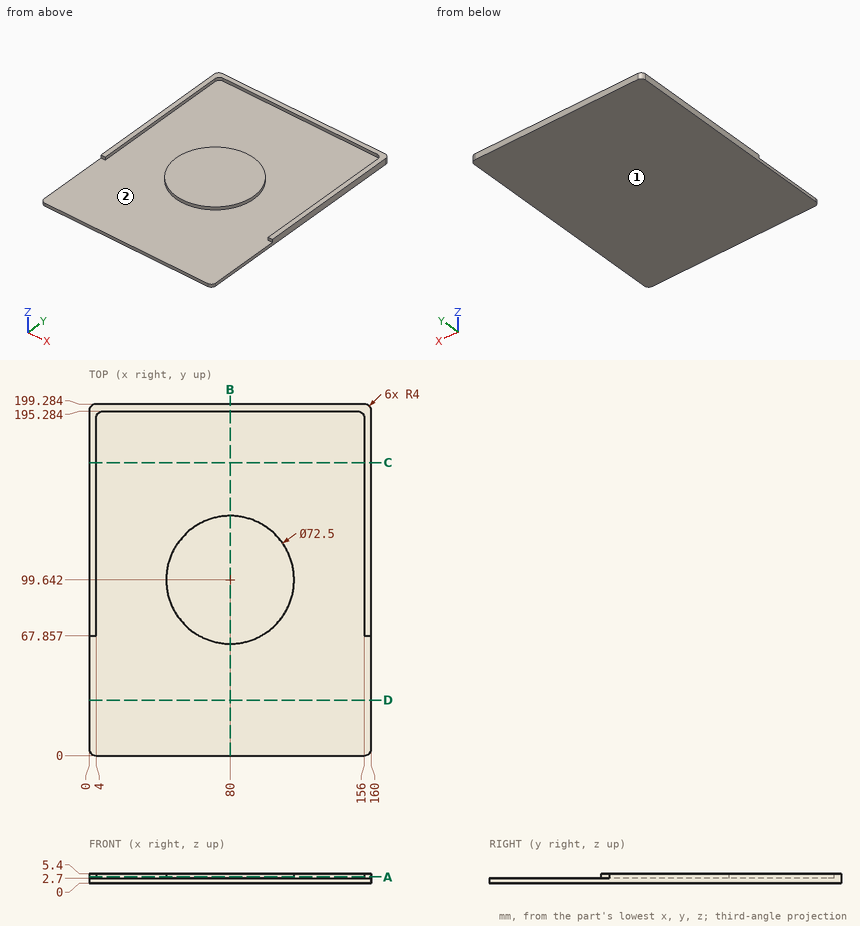
The figure shows three views and two pictorial views of one solid part (mm, origin at its lowest corner). Answer the questions. Round coordinates to 2 decimals unless told otherwise and drop trailing zeros. Loops run counter-clockwise (first coordinate to the right, second up) from the corner with the lowest first, then second, coordinate; pieces in that order, holes last. Notation, with made-up numbers: M 69,-23.75 L 89,-23.75 A19 ccw 89,-11.75 Z; hole C 20.5,-27 d4. An arc over 180 degrees is marked long. Write each question's results on one line, items separated by ' | '. Start each with the question number.
1) Find section B-B on x = 80. Write down the section's boundary in (y, z).
2) Each of these flat-tipped pins is pushed along its axis until it touches: pin 1 (1.4 mm diameter, centred on x = 68, z = 3.5, fed in from -Y); pin 2 (1.4 mm diameter, centred on x = 2, z = 4, fed in from -Y). Where does it stop, or does it pass through?
3) Find section C-C on y = 166. Write down the section's boundary in (x, z).
4) Find section A-A on z = 3.6. Write down the section's boundary in (x, y).
5) Find section D-D on y = 31.5. Write down the section's boundary in (x, z).
6) Determine the mould class of the marked faces 1 and 2 for opening direction X: pulls with the +X half, pulls with the -X half, needs draft (parallel to the pull), parting line crosses it, or undercut.
7) Straight lines are drawn through the part: probe 1 along X at (y, z) = (190.5, 3.35); probe 2 along X at (y, z) = (122, 2.75) (1 decimal); probe 3 along Z at (x, y) = (120.5, 116). For each, find the intervals that lie inside material, in ascending order.
Final values:
1) outline: M 0,0 L 199.28,0 L 199.28,5.4 L 195.28,5.4 L 195.28,2.7 L 135.89,2.7 L 135.89,5.4 L 63.39,5.4 L 63.39,2.7 L 0,2.7 Z
2) pin 1: y = 65.2 | pin 2: y = 67.86
3) outline: M 0,0 L 160,0 L 160,5.4 L 156,5.4 L 156,2.7 L 4,2.7 L 4,5.4 L 0,5.4 Z
4) outline: M 0,67.86 L 4,67.86 L 4,191.28 A4 cw 8,195.28 L 152,195.28 A4 cw 156,191.28 L 156,67.86 L 160,67.86 L 160,195.28 A4 ccw 156,199.28 L 4,199.28 A4 ccw 0,195.28 Z; C 80,99.64 d72.5
5) outline: M 0,0 L 160,0 L 160,2.7 L 0,2.7 Z
6) face 1: needs draft | face 2: undercut
7) probe 1: 0 to 4, 156 to 160 | probe 2: 0 to 4, 51.5 to 108.5, 156 to 160 | probe 3: 0 to 2.7
